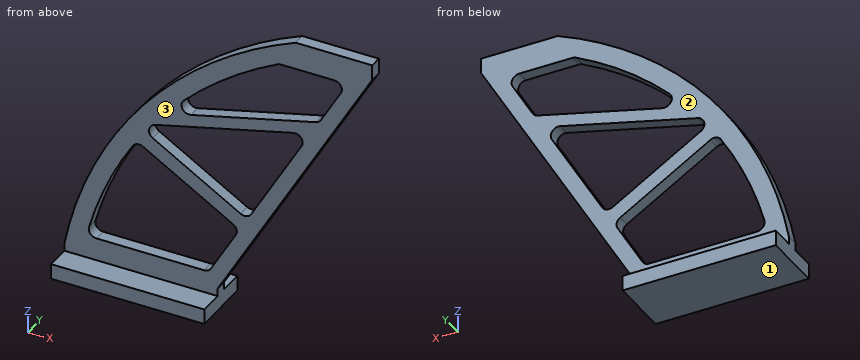
```python
from build123d import *

# Parameters (mm, degrees)
F1_DEPTH = 4.064
F0_W     = 101.6
F0_H     = 10.16
F2_DEPTH = 20.32


with BuildPart() as f1:
    # F0 (on Front) → F1 (new body, symmetric)
    with BuildSketch(Plane.XZ):
        with BuildLine():
            ThreePointArc((153.452878, 203.2), (52.830692, 128.728784), (0, 15.24))
            Line((0, 15.24), (0, 10.16))
            Line((0, 10.16), (101.6, 10.16))
            Line((101.6, 10.16), (101.6, 15.24))
            Line((101.6, 15.24), (204.252878, 193.04))
            Line((204.252878, 193.04), (204.252878, 203.2))
            Line((204.252878, 203.2), (153.452878, 203.2))
        make_face()
        with BuildLine():
            Line((92.801182, 25.4), (21.226424, 25.4))
            ThreePointArc((21.226424, 25.4), (17.188655, 27.397336), (16.325996, 31.818734))
            ThreePointArc((16.325996, 31.818734), (28.359119, 65.714775), (45.287139, 97.450871))
            ThreePointArc((45.287139, 97.450871), (48.39745, 99.67396), (52.177043, 99.098778))
            Line((52.177043, 99.098778), (111.956531, 63.523804))
            ThreePointArc((111.956531, 63.523804), (114.27411, 60.440693), (113.758037, 56.618337))
            Line((113.758037, 56.618337), (97.200591, 27.94))
            ThreePointArc((97.200591, 27.94), (95.341182, 26.080591), (92.801182, 25.4))
        make_face(mode=Mode.SUBTRACT)
        with BuildLine():
            Line((60.353951, 116.882829), (151.789779, 139.711306))
            ThreePointArc((151.789779, 139.711306), (157.076895, 137.840462), (157.419723, 132.242596))
            Line((157.419723, 132.242596), (123.918924, 74.21751))
            ThreePointArc((123.918924, 74.21751), (120.801871, 71.842028), (116.921611, 72.392043))
            Line((116.921611, 72.392043), (58.60911, 107.094008))
            ThreePointArc((58.60911, 107.094008), (56.220096, 110.491455), (57.164538, 114.535965))
            ThreePointArc((57.164538, 114.535965), (57.357158, 114.788721), (57.550111, 115.041224))
            ThreePointArc((57.550111, 115.041224), (58.795634, 116.200141), (60.353951, 116.882829))
        make_face(mode=Mode.SUBTRACT)
        with BuildLine():
            Line((143.720428, 184.912), (179.029599, 184.912))
            ThreePointArc((179.029599, 184.912), (183.429008, 182.372), (183.429008, 177.292))
            Line((183.429008, 177.292), (170.135294, 154.266611))
            ThreePointArc((170.135294, 154.266611), (168.793752, 152.75003), (166.966419, 151.877901))
            Line((166.966419, 151.877901), (84.043811, 131.174891))
            ThreePointArc((84.043811, 131.174891), (78.387658, 133.609547), (79.234455, 139.708936))
            ThreePointArc((79.234455, 139.708936), (108.561894, 164.521107), (141.448627, 184.375712))
            ThreePointArc((141.448627, 184.375712), (142.553307, 184.776111), (143.720428, 184.912))
        make_face(mode=Mode.SUBTRACT)
    extrude(amount=F1_DEPTH, both=True)

    # F0 (on Front) → F2 (join, symmetric)
    with BuildSketch(Plane.XZ):
        with Locations((50.8, 5.08)):
            Rectangle(F0_W, F0_H)
    extrude(amount=F2_DEPTH, both=True)


solid = f1.part
```
Design review of the part built by this model. Coordinates are the model's own, in mm. Face numbers are marked on the shaded views. A direction names the side the tool comes from. Coordinates: 2 decimals unless noted, no trailing zeros. Loops run counter-clockwise (first coordinate to the right, second up) from the corner with the lowest first, then second, coordinate; pieces in that order, holes last.
Q1. To check wall thickness, follow line 1 (Z direction, x = 16.5, y = 15); line 2 (X direction, y = -1.5, z = 31); line 3 (X direction, y = -3, z = 55). State the ranges of each line that lie inside material, in increasing order.
Reported:
line 1: z = 0 to 10.16
line 2: x = 3.5 to 16.17, 98.97 to 110.7
line 3: x = 10.92 to 23.93, 112.82 to 124.56
Q2. For pin 1 (12 mm diameter, centred on y = -6, z = 11, fed in from +X); pin 2 (6 mm diameter, centred on y = -3.5, z = 56.5, fed in from +X); pin 3 (1 mm diameter, centred on x = 32.5, z = 74.5, fed in from -Y), all flat-tipped, find the tip position at first contact; note any pin that passes through.
Reported:
pin 1: stops at x = 102.43
pin 2: stops at x = 127.15
pin 3: stops at y = -4.06
Q3. We need section A-A on z = 142.5. State the section outline as (x, y) points.
Reported:
outline: (64.93, -4.06) - (82.09, -4.06) - (82.09, 4.06) - (64.93, 4.06) - close; (129.4, -4.06) - (175.07, -4.06) - (175.07, 4.06) - (129.4, 4.06) - close
Q4. We need section C-C on x = 135. State the section outline as (y, z) points.
Reported:
outline: (-4.06, 73.09) - (4.06, 73.09) - (4.06, 93.41) - (-4.06, 93.41) - close; (-4.06, 135.52) - (4.06, 135.52) - (4.06, 143.9) - (-4.06, 143.9) - close; (-4.06, 181.03) - (4.06, 181.03) - (4.06, 194.78) - (-4.06, 194.78) - close
Q5. Tool access review of the marked faces 1, 2 and 3: name each direction out of +Z, -Z, +X, -X, +Y, -Y from which nothing blocks a thin tool from reaching the whole face with its end or side.
Reported:
face 1: -Z, +X, -X, +Y, -Y
face 2: +Z, +X, -X, +Y
face 3: +Z, +X, -X, -Y
Q6. We need section D-D on x = 27. State the section outline as (y, z) points, and give its area (3 significant figures).
Reported:
outline: (-20.32, 0) - (20.32, 0) - (20.32, 10.16) - (4.06, 10.16) - (4.06, 25.4) - (-4.06, 25.4) - (-4.06, 10.16) - (-20.32, 10.16) - close; (-4.06, 62.57) - (4.06, 62.57) - (4.06, 90.45) - (-4.06, 90.45) - close
area: 763 mm2
Q7. We need section B-B on y = -1. State how many separate pieces and enclosed holes the cut face has, and give its area (3 significant figures).
Reported:
separate pieces: 1
enclosed holes: 3
area: 10,100 mm2
